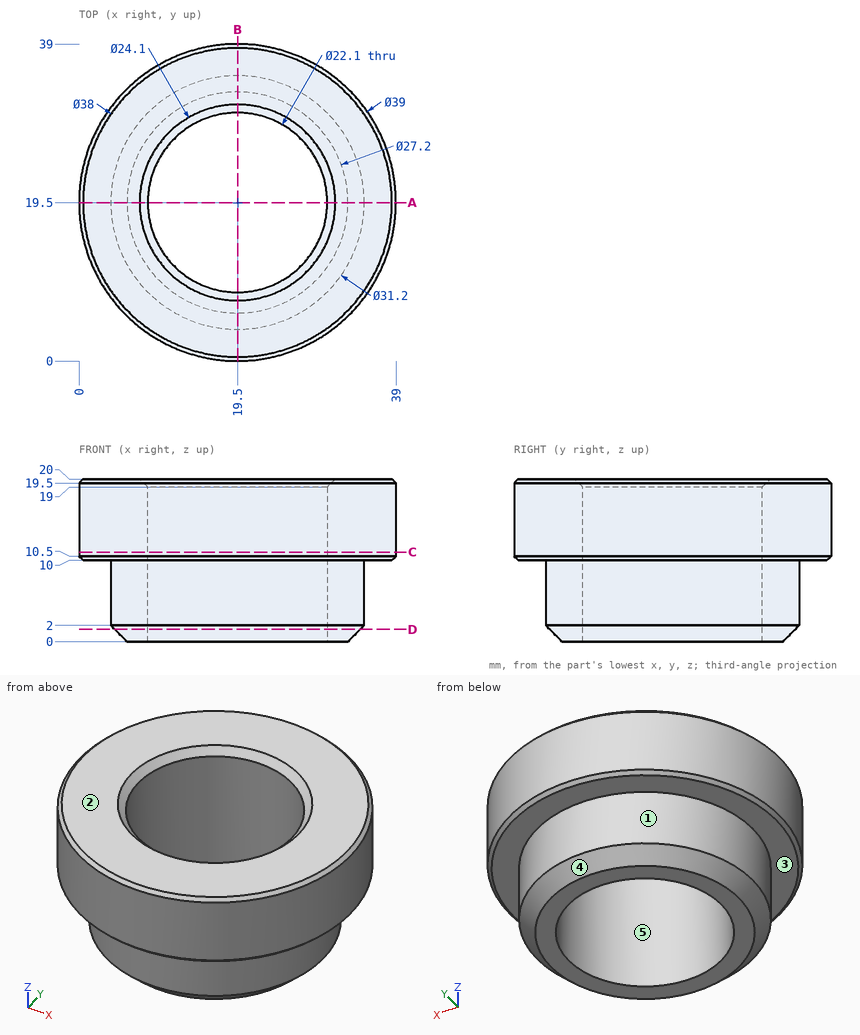
The figure shows three views and two pictorial views of one solid part (mm, origin at its lowest corner). Answer the questions. A direction names the side the tool comes from. Coordinates: 2 decimals unless noted, no trailing zeros. Write each loop counter-clockwise with the first axis right and the second up, starting at its lowest first coordinate (ties: lowest second). Pieces come first, ordered by that corner, then holes. Notation, with made-up numbers: M 31.5,41.5 L 56.5,41.5 A15 cw 56.5,69.5 Z; hole C 35.5,46.25 d5. An arc over 180 degrees is marked long. Answer as CSV lines item,"result". Start each with the question number.
Item 1: Determine the mould class of the marked faces 3, 4 and 5 for opening direction X: released by +X, released by -X, zero draft, split by the parting line, or undercut.
Item 2: Consider L1, parallel to Y at x = 19.5, z = 4; L2, parallel to Y at x = 19.5, z = 12.5; L3, parallel to X at y = 23, z = 17. Determine where each line is inside the solid, lowest interval first.
Item 3: A tool of negligible diameter and unlimited length cuts with its end or side. For the marked faces 1 and 2, from which of +Z, -Z, +X, -X, +Y, -Y can it reach the whole face along a straight path? Write none if from no direction.
Item 4: Flat-ended cylindrical pins translate along their axes: P1, Ø2, axis at y = 11.5, z = 13, coming from the +X side; P2, Ø12, axis at y = 30.5, z = 14.5, coming from the -X side; P3, Ø8, axis at x = 15.5, z = 10, coming from the +Y side. Find the tip coordinate at first contact, or state that the pin passes through.
Item 5: Section A-A on y = 19.5 is taken. Write down the section's boundary in (x, z), and give its area (4 significant figures).
Item 6: Section D-D on z = 1.5 is taken. Write down the section's boundary in (x, y).
Item 7: Section C-C on z = 11 is taken. Write down the section's boundary in (x, y), and give its area (3 significant figures).
Checks:
1,face 3,"zero draft"
1,face 4,"split by the parting line"
1,face 5,"undercut"
2,L1,"y = 3.9 to 8.45, 30.55 to 35.1"
2,L2,"y = 0 to 8.45, 30.55 to 39"
2,L3,"x = 0.32 to 9.02, 29.98 to 38.68"
3,face 1,"-Z"
3,face 2,"+Z, +X, -X, +Y, -Y"
4,P1,"stops at x = 37.7"
4,P2,"stops at x = 0.65"
4,P3,"stops at y = 39"
5,outline,"M 0,10.5 L 0.5,10 L 3.9,10 L 3.9,2 L 5.9,0 L 8.45,0 L 8.45,19 L 7.45,20 L 0.5,20 L 0,19.5 Z; M 30.55,0 L 33.1,0 L 35.1,2 L 35.1,10 L 38.5,10 L 39,10.5 L 39,19.5 L 38.5,20 L 31.55,20 L 30.55,19 Z"
5,area,"254.5 mm²"
6,outline,"C 19.5,19.5 d30.2; hole C 19.5,19.5 d22.1"
7,outline,"C 19.5,19.5 d39; hole C 19.5,19.5 d22.1"
7,area,"811 mm²"
